Could you check a few things on this drawing? It's one solid part, dimensions in mm from its lowest x, y, z. A direction names the side the tool comes from. Coordinates: 2 decimals unless noted, no trailing zeros. Write each loop counter-clockwise with the first axis right and the second up, starting at its lowest first coordinate (ties: lowest second). Pieces come first, ordered by that corner, then holes.
Item 1: I want a section at A-A (x = 15). Please give me the cut outline in (y, z), and give its area (3 significant figures).
Item 2: I'm going to push flat-ended pins straight in: P1, Ø11, axis at y = 31, z = 22.5, coming from the -X side; P2, Ø2, axis at x = 7.5, z = 34.5, coming from the -Y side; P3, Ø7.5, axis at y = 9, z = 29.5, coming from the -X side. Where does each tip first touch, or does it pass through?
Item 3: If we mould it in two halves opening along Y, with no side actions, what happens to the marked faces 1, 2 and 3? For each: pulls with the +Y half, pulls with the -Y half, needs draft (parallel to the pull), parting line crosses it, or undercut.
Item 4: I want a section at C-C (x = 31). Please give me the cut outline in (y, z).
Item 5: For the marked faces 4, 5 and 6, which set-ups out of +Z, -Z, +X, -X, +Y, -Y let a thin tool reach every point of the face, with its end or its side?
Item 6: Please list where these lines run through material, in increasing order: line 1 (Y direction, x = 17, z = 24); line 2 (Y direction, x = 33, z = 9); line 3 (X direction, y = 12.5, z = 29).
Item 7: I want a section at B-B (z = 16). Please give me the cut outline in (x, y).
Item 8: I want a section at D-D (y = 42.5). Please give me the cut outline in (x, z), and give its area (3 significant figures).
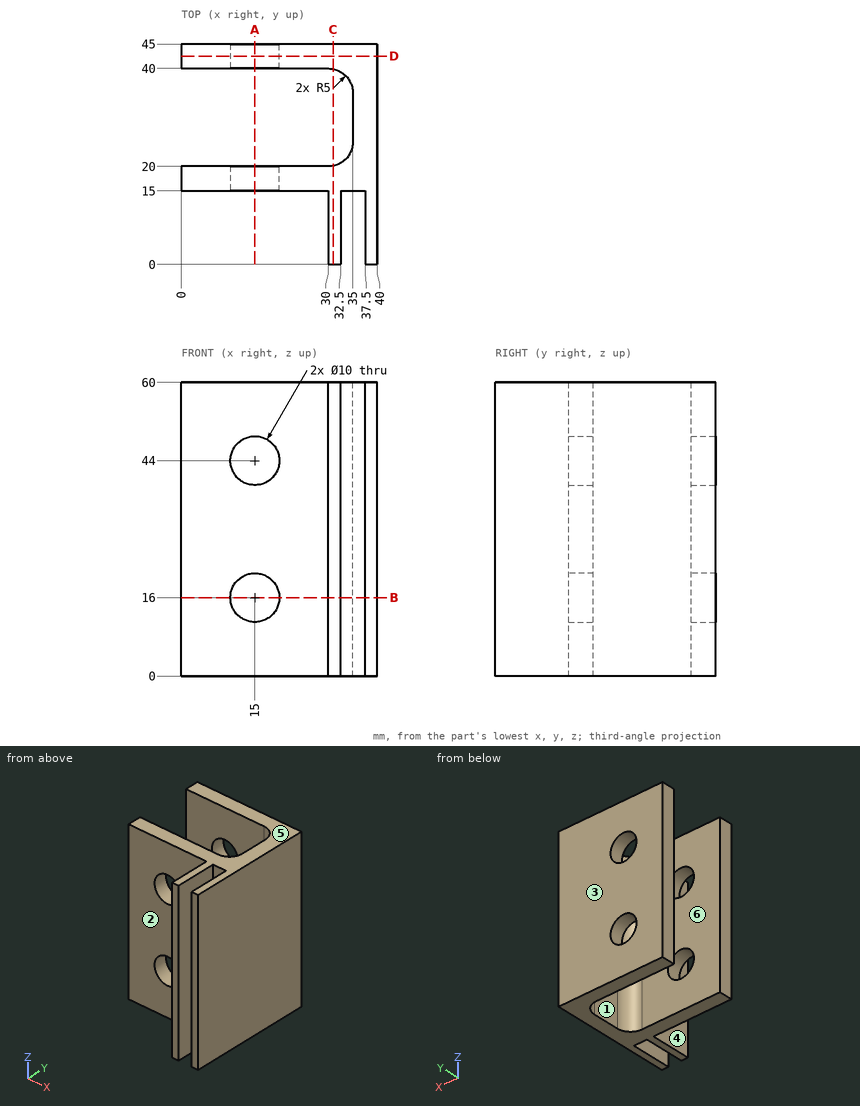
Answer:
1. outline: (15, 0) - (20, 0) - (20, 11) - (15, 11) - close; (15, 21) - (20, 21) - (20, 39) - (15, 39) - close; (15, 49) - (20, 49) - (20, 60) - (15, 60) - close; (40, 0) - (45, 0) - (45, 11) - (40, 11) - close; (40, 21) - (45, 21) - (45, 39) - (40, 39) - close; (40, 49) - (45, 49) - (45, 60) - (40, 60) - close
1. area: 400 mm2
2. P1: stops at x = 34.77
2. P2: stops at y = 15
2. P3: stops at x = 30
3. face 1: undercut
3. face 2: pulls with the -Y half
3. face 3: pulls with the +Y half
4. outline: (0, 0) - (20.1, 0) - (20.1, 60) - (0, 60) - close; (39.9, 0) - (45, 0) - (45, 60) - (39.9, 60) - close
5. face 4: +Z, -Z, -X, -Y
5. face 5: +Z, +X, -X, +Y, -Y
5. face 6: +Z, -Z, -X
6. line 1: y = 15 to 20, 40 to 45
6. line 2: y = 15 to 21, 39 to 45
6. line 3: x = 30 to 32.5, 37.5 to 40
7. outline: (0, 15) - (10, 15) - (10, 20) - (0, 20) - close; (0, 40) - (10, 40) - (10, 45) - (0, 45) - close; (20, 15) - (30, 15) - (30, 0) - (32.5, 0) - (32.5, 15) - (37.5, 15) - (37.5, 0) - (40, 0) - (40, 45) - (20, 45) - (20, 40) - (30, 40) arc R5 cw to (35, 35) - (35, 25) arc R5 cw to (30, 20) - (20, 20) - close
8. outline: (0, 0) - (40, 0) - (40, 60) - (0, 60) - close; hole circle Ø10 at (15, 16); hole circle Ø10 at (15, 44)
8. area: 2,240 mm2
